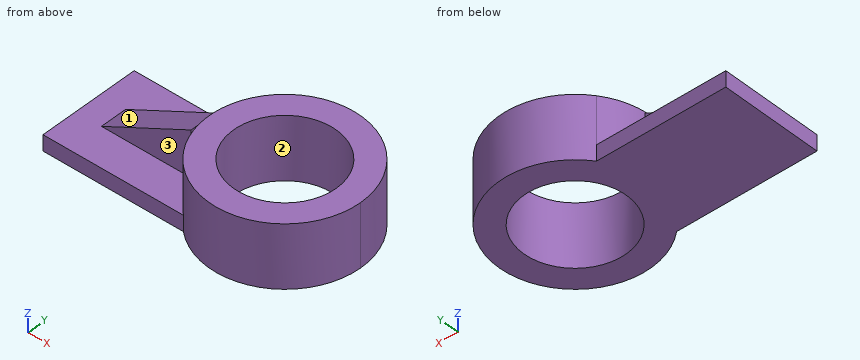
from build123d import *

# Parameters (mm, degrees)
F1_DEPTH = 6.35
F0_R     = 20.703057
F2_DEPTH = 25.4
F4_DEPTH = 18.542
F6_DEPTH = 25.4


with BuildPart() as f1:
    # F0 (on Top) → F1 (new body)
    with BuildSketch(Plane.XY):
        with BuildLine():
            ThreePointArc((24.584481, -6.386341), (14.495983, 13.150341), (20.096751, 34.412776))
            Line((20.096751, 34.412776), (-32.172695, 34.412776))
            Line((-32.172695, 34.412776), (-32.172695, -6.386341))
            Line((-32.172695, -6.386341), (24.584481, -6.386341))
        make_face()
    extrude(amount=F1_DEPTH)

    # F0 (on Top) → F2 (join)
    with BuildSketch(Plane.XY):
        with BuildLine():
            ThreePointArc((24.584481, -6.386341), (57.484915, -11.444852), (75.572235, 16.499306))
            ThreePointArc((75.572235, 16.499306), (54.354409, 45.647298), (20.096751, 34.412776))
            ThreePointArc((20.096751, 34.412776), (14.495983, 13.150341), (24.584481, -6.386341))
        make_face()
        with Locations((44.942293, 16.499306)):
            Circle(F0_R, mode=Mode.SUBTRACT)
    extrude(amount=F2_DEPTH)

    # F3 (on face) → F4 (join)
    with BuildSketch(Plane.XY.offset(6.35)):
        with BuildLine():
            ThreePointArc((14.423249, 13.89521), (14.312351, 16.499306), (14.423249, 19.103403))
            Line((14.423249, 19.103403), (-21.812018, 19.103403))
            Line((-21.812018, 19.103403), (-21.812018, 8.304046))
            Line((-21.812018, 8.304046), (14.423249, 8.304046))
            Line((14.423249, 8.304046), (14.423249, 13.89521))
        make_face()
    extrude(amount=F4_DEPTH)

    # F5 (on face) → F6 (cut)
    with BuildSketch(Plane.XZ.offset(-8.304046)):
        Polygon((-21.812018, 24.892), (-21.812018, 6.35), (14.423249, 24.892), align=None)
    extrude(amount=-F6_DEPTH, mode=Mode.SUBTRACT)


solid = f1.part
Geometry: final body of the model. Coordinates: model frame, mm. Face numbers are marked on the shaded views. Give positions to 0.01 mm unless a question says otherwise; leave off trailing zeros. Write each loop counter-clockwise with the first axis right and the second up, starting at its lowest first coordinate (ties: lowest second). Pieces come first, ordered by that corner, then holes.
(1) First-contact query: P1, Ø10, axis at y = 34.5, z = 22, coming from the +X side; P2, Ø1, axis at x = 32, z = 22, coming from the +Y side; P3, Ø1.5, axis at x = -12, y = 35, coming from the +Z side. Flat tips, straight axial feed; report the tip coordinate or a pass-through.
(2) Cut plane A-A, the plane z = 3. Return loops of the section in (x, y).
(3) Cut plane D-D, the plane x = -23.5. Return loops of the section in (y, z), then the cut area to 3 significant figures.
(4) Ray query, line 1 (X direction, y = 12.5, z = 8); line 2 (Y direction, x = 54.5, z = 8.25); line 3 (Z direction, x = -15, y = 31.5). Return the intervals inside material, ascending.
(5) Cut plane C-C, the plane x = 28. Return loops of the section in (y, z), then the cut area to 3 significant figures.
(6) Cut plane B-B, the plane y = 18. Return loops of the section in (x, z), then the cut area to 3 significant figures.
(7) Mould query, pull axis X, two halves, no side actions, for the marked faces 1, 2 and 3. Classes: released by +X, released by -X, zero draft, split by the parting line, or undercut.
Values follow:
1. P1: stops at x = 72.68
1. P2: stops at y = 44.49
1. P3: stops at z = 6.35
2. outline: (-32.17, -6.39) - (24.58, -6.39) arc R30.63 ccw (long way) to (20.1, 34.41) - (-32.17, 34.41) - close; hole circle Ø41.41 at (44.94, 16.5)
3. outline: (-6.39, 0) - (34.41, 0) - (34.41, 6.35) - (-6.39, 6.35) - close
3. area: 259 mm2
4. line 1: x = -18.59 to 14.42, 14.57 to 24.63, 65.26 to 75.31
4. line 2: y = -12.6 to -1.87, 34.86 to 45.6
4. line 3: z = 0 to 6.35
5. outline: (-9.02, 0) - (4.6, 0) - (4.6, 25.4) - (-9.02, 25.4) - close; (28.4, 0) - (42.02, 0) - (42.02, 25.4) - (28.4, 25.4) - close
5. area: 692 mm2
6. outline: (-32.17, 0) - (24.29, 0) - (24.29, 25.4) - (14.35, 25.4) - (14.35, 24.89) - (14.42, 24.89) - (-21.81, 6.35) - (-32.17, 6.35) - close; (65.59, 0) - (75.54, 0) - (75.54, 25.4) - (65.59, 25.4) - close
6. area: 1,140 mm2
7. face 1: released by -X
7. face 2: undercut
7. face 3: zero draft
